Build history of the part. All positions in model axes, mm. Coordinates: 2 decimals unless noted, no trailing zeros. Order: outer loops, then holes, each group sorted by start corner. A loop starts at its lowest first (then second) coordinate and runs counter-clockwise, first axis right, second up. Notation, with made-up numbers: (61.5, 59.5) - (102.5, 59.5) arc R25 ccw to (102.5, 87.5) - close; hole circle Ø7 at (-2, 6.5). An arc over 180 degrees is marked (long way). One line per item, written item: value.
from build123d import *

# Parameters (mm, degrees)
ESQUISSE1_R        = 3.4
BOSS_EXTRU_1_DEPTH = 400


with BuildPart() as part:
    # Esquisse1 → Boss.-Extru.1 (new body)
    with BuildSketch(Plane(origin=(0, 0, -30), x_dir=(-1, 0, 0), z_dir=(0, 0, -1))):
        with BuildLine():
            Line((-4.5, 15), (-4.5, 13.5))
            ThreePointArc((-4.5, 13.5), (-4.353553391, 13.146446609), (-4, 13))
            Line((-4, 13), (-2.5, 13))
            ThreePointArc((-2.5, 13), (-2.146446609, 12.853553391), (-2, 12.5))
            ThreePointArc((-2, 12.5), (-2.732233047, 10.732233047), (-4.5, 10))
            Line((-4.5, 10), (-5.807611845, 10))
            ThreePointArc((-5.807611845, 10), (-7.721029006, 10.380602337), (-9.343145751, 11.464466094))
            Line((-9.343145751, 11.464466094), (-10.785533906, 12.906854249))
            ThreePointArc((-10.785533906, 12.906854249), (-11.869397663, 14.528970994), (-12.25, 16.442388155))
            Line((-12.25, 16.442388155), (-12.25, 23.557611845))
            ThreePointArc((-12.25, 23.557611845), (-11.869397663, 25.471029006), (-10.785533906, 27.093145751))
            Line((-10.785533906, 27.093145751), (-9.343145751, 28.535533906))
            ThreePointArc((-9.343145751, 28.535533906), (-7.721029006, 29.619397663), (-5.807611845, 30))
            Line((-5.807611845, 30), (-4.5, 30))
            ThreePointArc((-4.5, 30), (-2.732233047, 29.267766953), (-2, 27.5))
            ThreePointArc((-2, 27.5), (-2.146446609, 27.146446609), (-2.5, 27))
            Line((-2.5, 27), (-4, 27))
            ThreePointArc((-4, 27), (-4.353553391, 26.853553391), (-4.5, 26.5))
            Line((-4.5, 26.5), (-4.5, 25))
            ThreePointArc((-4.5, 25), (-4.207106781, 24.292893219), (-3.5, 24))
            Line((-3.5, 24), (-1.5, 24))
            ThreePointArc((-1.5, 24), (-0.439339828, 24.439339828), (0, 25.5))
            Line((0, 25.5), (0, 36))
            ThreePointArc((0, 36), (-1.171572875, 38.828427125), (-4, 40))
            Line((-4, 40), (-14.5, 40))
            ThreePointArc((-14.5, 40), (-15.560660172, 39.560660172), (-16, 38.5))
            Line((-16, 38.5), (-16, 36.5))
            ThreePointArc((-16, 36.5), (-15.707106781, 35.792893219), (-15, 35.5))
            Line((-15, 35.5), (-13.5, 35.5))
            ThreePointArc((-13.5, 35.5), (-13.146446609, 35.646446609), (-13, 36))
            Line((-13, 36), (-13, 37.5))
            ThreePointArc((-13, 37.5), (-12.853553391, 37.853553391), (-12.5, 38))
            ThreePointArc((-12.5, 38), (-10.732233047, 37.267766953), (-10, 35.5))
            Line((-10, 35.5), (-10, 34.192388155))
            ThreePointArc((-10, 34.192388155), (-10.380602337, 32.278970994), (-11.464466094, 30.656854249))
            Line((-11.464466094, 30.656854249), (-12.906854249, 29.214466094))
            ThreePointArc((-12.906854249, 29.214466094), (-14.528970994, 28.130602337), (-16.442388155, 27.75))
            Line((-16.442388155, 27.75), (-23.557611845, 27.75))
            ThreePointArc((-23.557611845, 27.75), (-25.471029006, 28.130602337), (-27.093145751, 29.214466094))
            Line((-27.093145751, 29.214466094), (-28.535533906, 30.656854249))
            ThreePointArc((-28.535533906, 30.656854249), (-29.619397663, 32.278970994), (-30, 34.192388155))
            Line((-30, 34.192388155), (-30, 35.5))
            ThreePointArc((-30, 35.5), (-29.267766953, 37.267766953), (-27.5, 38))
            ThreePointArc((-27.5, 38), (-27.146446609, 37.853553391), (-27, 37.5))
            Line((-27, 37.5), (-27, 36))
            ThreePointArc((-27, 36), (-26.853553391, 35.646446609), (-26.5, 35.5))
            Line((-26.5, 35.5), (-25, 35.5))
            ThreePointArc((-25, 35.5), (-24.292893219, 35.792893219), (-24, 36.5))
            Line((-24, 36.5), (-24, 38.5))
            ThreePointArc((-24, 38.5), (-24.439339828, 39.560660172), (-25.5, 40))
            Line((-25.5, 40), (-36, 40))
            ThreePointArc((-36, 40), (-38.828427125, 38.828427125), (-40, 36))
            Line((-40, 36), (-40, 25.5))
            ThreePointArc((-40, 25.5), (-39.560660172, 24.439339828), (-38.5, 24))
            Line((-38.5, 24), (-36.5, 24))
            ThreePointArc((-36.5, 24), (-35.792893219, 24.292893219), (-35.5, 25))
            Line((-35.5, 25), (-35.5, 26.5))
            ThreePointArc((-35.5, 26.5), (-35.646446609, 26.853553391), (-36, 27))
            Line((-36, 27), (-37.5, 27))
            ThreePointArc((-37.5, 27), (-37.853553391, 27.146446609), (-38, 27.5))
            ThreePointArc((-38, 27.5), (-37.267766953, 29.267766953), (-35.5, 30))
            Line((-35.5, 30), (-34.192388155, 30))
            ThreePointArc((-34.192388155, 30), (-32.278970994, 29.619397663), (-30.656854249, 28.535533906))
            Line((-30.656854249, 28.535533906), (-29.214466094, 27.093145751))
            ThreePointArc((-29.214466094, 27.093145751), (-28.130602337, 25.471029006), (-27.75, 23.557611845))
            Line((-27.75, 23.557611845), (-27.75, 16.442388155))
            ThreePointArc((-27.75, 16.442388155), (-28.130602337, 14.528970994), (-29.214466094, 12.906854249))
            Line((-29.214466094, 12.906854249), (-30.656854249, 11.464466094))
            ThreePointArc((-30.656854249, 11.464466094), (-32.278970994, 10.380602337), (-34.192388155, 10))
            Line((-34.192388155, 10), (-35.5, 10))
            ThreePointArc((-35.5, 10), (-37.267766953, 10.732233047), (-38, 12.5))
            ThreePointArc((-38, 12.5), (-37.853553391, 12.853553391), (-37.5, 13))
            Line((-37.5, 13), (-36, 13))
            ThreePointArc((-36, 13), (-35.646446609, 13.146446609), (-35.5, 13.5))
            Line((-35.5, 13.5), (-35.5, 15))
            ThreePointArc((-35.5, 15), (-35.792893219, 15.707106781), (-36.5, 16))
            Line((-36.5, 16), (-38.5, 16))
            ThreePointArc((-38.5, 16), (-39.560660172, 15.560660172), (-40, 14.5))
            Line((-40, 14.5), (-40, 4))
            ThreePointArc((-40, 4), (-38.828427125, 1.171572875), (-36, 0))
            Line((-36, 0), (-25.5, 0))
            ThreePointArc((-25.5, 0), (-24.439339828, 0.439339828), (-24, 1.5))
            Line((-24, 1.5), (-24, 3.5))
            ThreePointArc((-24, 3.5), (-24.292893219, 4.207106781), (-25, 4.5))
            Line((-25, 4.5), (-26.5, 4.5))
            ThreePointArc((-26.5, 4.5), (-26.853553391, 4.353553391), (-27, 4))
            Line((-27, 4), (-27, 2.5))
            ThreePointArc((-27, 2.5), (-27.146446609, 2.146446609), (-27.5, 2))
            ThreePointArc((-27.5, 2), (-29.267766953, 2.732233047), (-30, 4.5))
            Line((-30, 4.5), (-30, 5.807611845))
            ThreePointArc((-30, 5.807611845), (-29.619397663, 7.721029006), (-28.535533906, 9.343145751))
            Line((-28.535533906, 9.343145751), (-27.093145751, 10.785533906))
            ThreePointArc((-27.093145751, 10.785533906), (-25.471029006, 11.869397663), (-23.557611845, 12.25))
            Line((-23.557611845, 12.25), (-16.442388155, 12.25))
            ThreePointArc((-16.442388155, 12.25), (-14.528970994, 11.869397663), (-12.906854249, 10.785533906))
            Line((-12.906854249, 10.785533906), (-11.464466094, 9.343145751))
            ThreePointArc((-11.464466094, 9.343145751), (-10.380602337, 7.721029006), (-10, 5.807611845))
            Line((-10, 5.807611845), (-10, 4.5))
            ThreePointArc((-10, 4.5), (-10.732233047, 2.732233047), (-12.5, 2))
            ThreePointArc((-12.5, 2), (-12.853553391, 2.146446609), (-13, 2.5))
            Line((-13, 2.5), (-13, 4))
            ThreePointArc((-13, 4), (-13.146446609, 4.353553391), (-13.5, 4.5))
            Line((-13.5, 4.5), (-15, 4.5))
            ThreePointArc((-15, 4.5), (-15.707106781, 4.207106781), (-16, 3.5))
            Line((-16, 3.5), (-16, 1.5))
            ThreePointArc((-16, 1.5), (-15.560660172, 0.439339828), (-14.5, 0))
            Line((-14.5, 0), (-4, 0))
            ThreePointArc((-4, 0), (-1.171572875, 1.171572875), (0, 4))
            Line((0, 4), (0, 14.5))
            ThreePointArc((0, 14.5), (-0.439339828, 15.560660172), (-1.5, 16))
            Line((-1.5, 16), (-3.5, 16))
            ThreePointArc((-3.5, 16), (-4.207106781, 15.707106781), (-4.5, 15))
        make_face()
        with Locations(Location((-20, 20, 0), (0, 0, 180))):
            Circle(ESQUISSE1_R, mode=Mode.SUBTRACT)
        with BuildLine():
            Line((-4, 1.8), (-7.7, 1.8))
            ThreePointArc((-7.7, 1.8), (-8.053553391, 1.946446609), (-8.2, 2.3))
            Line((-8.2, 2.3), (-8.2, 7.7))
            ThreePointArc((-8.2, 7.7), (-8.053553391, 8.053553391), (-7.7, 8.2))
            Line((-7.7, 8.2), (-2.3, 8.2))
            ThreePointArc((-2.3, 8.2), (-1.946446609, 8.053553391), (-1.8, 7.7))
            Line((-1.8, 7.7), (-1.8, 4))
            ThreePointArc((-1.8, 4), (-2.444365081, 2.444365081), (-4, 1.8))
        make_face(mode=Mode.SUBTRACT)
        with BuildLine():
            Line((-38.2, 4), (-38.2, 7.7))
            ThreePointArc((-38.2, 7.7), (-38.053553391, 8.053553391), (-37.7, 8.2))
            Line((-37.7, 8.2), (-32.3, 8.2))
            ThreePointArc((-32.3, 8.2), (-31.946446609, 8.053553391), (-31.8, 7.7))
            Line((-31.8, 7.7), (-31.8, 2.3))
            ThreePointArc((-31.8, 2.3), (-31.946446609, 1.946446609), (-32.3, 1.8))
            Line((-32.3, 1.8), (-36, 1.8))
            ThreePointArc((-36, 1.8), (-37.555634919, 2.444365081), (-38.2, 4))
        make_face(mode=Mode.SUBTRACT)
        with BuildLine():
            Line((-36, 38.2), (-32.3, 38.2))
            ThreePointArc((-32.3, 38.2), (-31.946446609, 38.053553391), (-31.8, 37.7))
            Line((-31.8, 37.7), (-31.8, 32.3))
            ThreePointArc((-31.8, 32.3), (-31.946446609, 31.946446609), (-32.3, 31.8))
            Line((-32.3, 31.8), (-37.7, 31.8))
            ThreePointArc((-37.7, 31.8), (-38.053553391, 31.946446609), (-38.2, 32.3))
            Line((-38.2, 32.3), (-38.2, 36))
            ThreePointArc((-38.2, 36), (-37.555634919, 37.555634919), (-36, 38.2))
        make_face(mode=Mode.SUBTRACT)
        with BuildLine():
            Line((-1.8, 36), (-1.8, 32.3))
            ThreePointArc((-1.8, 32.3), (-1.946446609, 31.946446609), (-2.3, 31.8))
            Line((-2.3, 31.8), (-7.7, 31.8))
            ThreePointArc((-7.7, 31.8), (-8.053553391, 31.946446609), (-8.2, 32.3))
            Line((-8.2, 32.3), (-8.2, 37.7))
            ThreePointArc((-8.2, 37.7), (-8.053553391, 38.053553391), (-7.7, 38.2))
            Line((-7.7, 38.2), (-4, 38.2))
            ThreePointArc((-4, 38.2), (-2.444365081, 37.555634919), (-1.8, 36))
        make_face(mode=Mode.SUBTRACT)
    extrude(amount=-BOSS_EXTRU_1_DEPTH)


solid = part.part
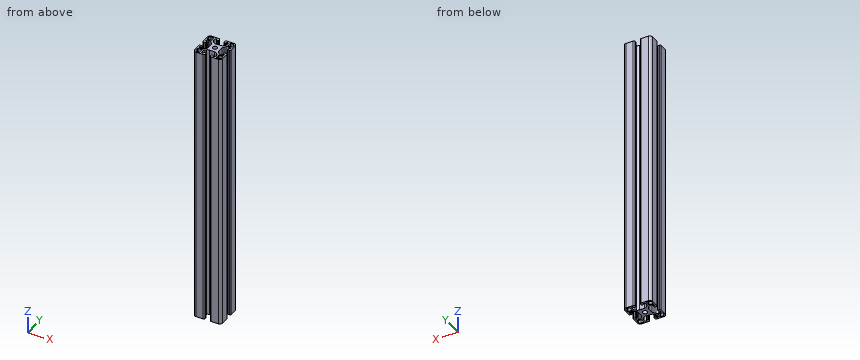
1. Flat gauge pins, fed straight in: P1, Ø2, axis at x = 20.5, z = 94, coming from the -Y side; P2, Ø1.6, axis at x = 37, z = 187.5, coming from the +Y side (3 decimals); P3, Ø1.6, axis at x = 38, z = 266, coming from the -Y side. Where does each tip first touch, or does it go through?
Values found:
P1: stops at y = 12.25
P2: stops at y = 39.995
P3: stops at y = 0.18
2. Band-saw the part on C-C, the plane z = 50. Count the separate pieces of the cut face and the enclosed holes in it, and give its area (3 significant figures).
Values found:
separate pieces: 1
enclosed holes: 5
area: 657 mm2
3. Probe line 1 along Y through (x, z) = (35, 265); line 2 along X through (y, z) = (33.5, 23.5); line 3 along X through (y, z) = (12.5, 160). List the from-to ranges inside material, lowest first.
Values found:
line 1: y = 0 to 1.8, 8.2 to 10, 30 to 31.8, 38.2 to 40
line 2: x = 0 to 1.8, 8.2 to 10.05, 29.95 to 31.8, 38.2 to 40
line 3: x = 0 to 2, 10.38 to 29.62, 38 to 40
4. Band-saw the part on A-A, the plane x = 20. Give the cut face in (y, z), and give its area (3 significant figures).
Values found:
outline: (12.25, -30) - (16.6, -30) - (16.6, 370) - (12.25, 370) - close; (23.4, -30) - (27.75, -30) - (27.75, 370) - (23.4, 370) - close
area: 3,480 mm2
